Autodesk Inventor part; units mm, degrees
ref_plane "YZ Plane" through (0, 0, 0) normal (1, 0, 0) x (0, 1, 0)
ref_plane "XZ Plane" through (0, 0, 0) normal (0, 1, 0) x (-1, 0, 0)
ref_plane "XY Plane" through (0, 0, 0) normal (0, 0, 1) x (1, 0, 0)
sketch "Boceto1" plane through (0, 0, 0) normal (0, 1, 0) x (-1, 0, 0)
  line L0 (40, 11) -> (40, 29.5)
  line L1 (40, 29.5) -> (0, 29.5)
  line L2 (0, 29.5) -> (0, 7.5)
  circle A0 centre (20, 12.5) radius 9.5
  line L3 (40, 11) -> (40, 1.5)
  line L4 (40, 1.5) -> (32, 1.5)
  line L5 (0, 7.5) -> (0, 1.5)
  line L6 (0, 1.5) -> (8, 1.5)
  line L7 (32, 1.5) -> (32, -5.5)
  line L8 (32, -5.5) -> (8, -5.5)
  line L9 (8, -5.5) -> (8, 1.5)
  point P0 (0, 0)
  point P1 (0, 0)
  dimension "d1" = 19
  dimension "d14" = 40
  dimension "d18" = 8
  dimension "d19" = 8
  dimension "d20" = 28
  dimension "d21" = 35
  dimension "d35" = 17
  dimension "d68" = 28
extrude "Extrusión1" add sketch "Boceto1" along normal blind 28
sketch "Boceto7" plane through (0, 0, 1.5) normal (0, 0, -1) x (-1, 0, 0)
  line L0 (0, 0) -> (0, 28)
  line L1 (0, 0) -> (4, 0)
  line L2 (40, 0) -> (0, 0)
  line L3 (4, 0) -> (4, 28)
  line L4 (40, 28) -> (0, 28)
  line L5 (4, 14) -> (4, 5)
  circle A0 centre (4, 5) radius 2
  circle A1 centre (4, 23) radius 2
  line L6 (40, 0) -> (40, 28)
  line L7 (40, 0) -> (36, 0)
  line L8 (36, 0) -> (36, 28)
  circle A2 centre (36, 5) radius 2
  circle A3 centre (36, 23) radius 2
  dimension "d24" = 4
  dimension "d25" = 4
  dimension "d26" = 5
  dimension "d27" = 5
  dimension "d28" = 4
  dimension "d29" = 4
  dimension "d30" = 4
  dimension "d31" = 5
  dimension "d32" = 5
  dimension "d60" = 4
extrude "Extrusión4" cut sketch "Boceto7" against normal blind 28 contours A0 L3 | L3 A0 | A1 L3 | L3 A1 | A2 L8 | L8 A2 | A3 L8 | L8 A3
sketch "Boceto9" plane through (0, 28, 0) normal (0, 1, 0) x (1, 0, 0)
  circle A0 centre (-20, -12.5) radius 9.5
  circle A1 centre (-8, -12.5) radius 1.5
  circle A2 centre (-32, -12.5) radius 1.5
  point P0 (0, 0)
  dimension "d36" = 12
  dimension "d38" = 3
  dimension "d39" = 3
  dimension "d61" = 12
sketch "Boceto10" plane through (0, 0, 0) normal (0, -1, 0) x (1, 0, 0)
  circle A0 centre (-20, 12.5) radius 9.5
  line L0 (-20, 12.5) -> (-8, 12.5)
  line L1 (-8, 12.5) -> (-32, 12.5)
  circle A1 centre (-32, 12.5) radius 1.5
  circle A2 centre (-8, 12.5) radius 1.5
  point P0 (0, 0)
  dimension "d40" = 12
  dimension "d41" = 24
  dimension "d42" = 3
  dimension "d43" = 3
hole "Agujero1" at (-32, 0, 12.5) at (-8, 0, 12.5) direction (0, 1, 0) diameter 3 depth 12.5 tip angle 118
hole "Agujero2" at (-8, 28, 12.5) at (-32, 28, 12.5) direction (0, -1, 0) diameter 3 depth 12.5 tip angle 118
thread "Rosca1"
thread "Rosca2"
thread "Rosca3"
thread "Rosca4"
equation "\"d68\" = d20"
properties part number "Soporte de Buje" material "Aluminum 6061"
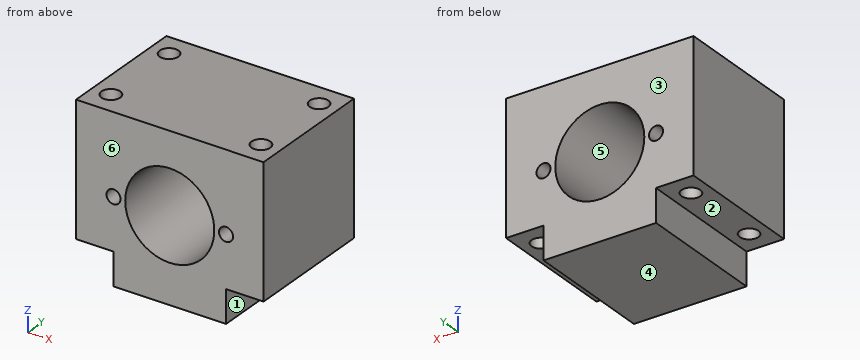
Check sheet for the modelled part. Datum: model origin and axes. Units: mm. Face numbers are marked on the shaded views. A direction names the side the tool comes from. Round coordinates to 2 decimals unless told otherwise and drop trailing zeros. Write each loop counter-clockwise with the first axis right and the second up, starting at its lowest first coordinate (ties: lowest second). Pieces come first, ordered by that corner, then holes. Notation, with made-up numbers: (-30, 51) - (24, 51) arc R11 ccw to (24, 64) - close; hole circle Ø2 at (34, 58). An arc over 180 degrees is marked (long way). Return JSON: item names as keys, results as strings.
Q1. Depth check by flat-ended pin: P1, Ø5.5, axis at y = 12, z = -1.5, coming from the +X side; P2, Ø4, axis at y = 7.5, z = 18.5, coming from the +X side; P3, Ø2.5, axis at x = -3, y = 17, coming from the -Z side; P4, Ø2.5, axis at x = -32, z = 12.5, coming from the -Y side. Enter the tip coordinate at first touch or a pass-through.
Returned:
{"P1": "stops at x = -8", "P2": "stops at x = 0", "P3": "stops at z = 1.5", "P4": "stops at y = 12.65"}
Q2. Access from +Z, -Z, +X, -X, +Y, -Y to the whole of each face (thin tool, end or side, straight path). Record for the marked faces 1, 2 and 3.
Returned:
{"face 1": "-Z, +X, +Y, -Y", "face 2": "-Z, -X, +Y, -Y", "face 3": "+Z, -Z, +X, -X, +Y"}
Q3. Cross-section at B-B (x = -36). Record the boundary of the cut face in (y, z).
Returned:
{"outline": "(0, 1.5) - (3, 1.5) - (3, 29.5) - (0, 29.5) - close; (7, 1.5) - (21, 1.5) - (21, 29.5) - (7, 29.5) - close; (25, 1.5) - (28, 1.5) - (28, 29.5) - (25, 29.5) - close"}
Q4. Cross-section at D-D (x = -20). Record the boundary of the cut face in (y, z), then the cut area to 3 significant figures.
Returned:
{"outline": "(0, -5.5) - (28, -5.5) - (28, 3) - (0, 3) - close; (0, 22) - (28, 22) - (28, 29.5) - (0, 29.5) - close", "area": "448 mm²"}
Q5. Scan lines: L1, parallel to Y at x = -4, z = 28.5; L2, parallel to X at y = 24.25, z = 20.5; L3, parallel to Y at x = -5, z = 21. Record each from-to range of solid material in increasing order. Write a range as from..to.
Returned:
{"L1": "y = 0..3, 7..21, 25..28", "L2": "x = -40..-37.56, -34.44..-25.12, -14.88..-5.56, -2.44..0", "L3": "y = 0..3.27, 6.73..21.27, 24.73..28"}
Q6. Draft check along Z on the marked faces 4, 5 and 6. Enter one of: released by +Z, released by -Z, zero draft, split by the parting line, or undercut.
Returned:
{"face 4": "released by -Z", "face 5": "undercut", "face 6": "zero draft"}
Q7. Cross-section at A-A (y = 23). Record the boundary of the cut face in (x, z), then the cut area to 3 significant figures.
Returned:
{"outline": "(-40, 1.5) - (-38, 1.5) - (-38, 29.5) - (-40, 29.5) - close; (-34, 1.5) - (-32, 1.5) - (-32, -5.5) - (-8, -5.5) - (-8, 1.5) - (-6, 1.5) - (-6, 29.5) - (-34, 29.5) - close; (-2, 1.5) - (0, 1.5) - (0, 29.5) - (-2, 29.5) - close; hole circle Ø3 at (-32, 12.5); hole circle Ø19 at (-20, 12.5); hole circle Ø3 at (-8, 12.5)", "area": "766 mm²"}
Q8. Cross-section at C-C (z = 9.5). Record the boundary of the cut face in (x, y).
Returned:
{"outline": "(-40, 0) - (-29.01, 0) - (-29.01, 28) - (-40, 28) - close; (-10.99, 0) - (0, 0) - (0, 28) - (-10.99, 28) - close; hole circle Ø4 at (-36, 5); hole circle Ø4 at (-36, 23); hole circle Ø4 at (-4, 5); hole circle Ø4 at (-4, 23)"}
